Study the drawing (mm; zero at the part's minimum x, y, z) and answer. A direction names the side the tool comes from. Round coordinates to 2 decimals unless told otherwise and drop trailing zeros. Write each loop counter-clockwise with the first axis right and the second up, starting at its lowest first coordinate (ties: lowest second). Pieces come first, ordered by that corner, then holes. Notation, with made-up numbers: (42.5, -29) - (71.5, -29) arc R12 ccw to (71.5, -8) - close; hole circle Ø8 at (-13.5, 40). An arc over 180 degrees is marked (long way). Use one line per item in the form item = value. Start each with the question number.
1) The part is cut by section C-C, the plane z = 7. Give the vertices of the cut face in (x, y).
2) This flat-tipped pin is pushed along its axis until it touches: pin 1 (24 mm diameter, centred on x = 157.5, y = 37.5, fed in from +Z). Where does it stop, or does it pass through?
3) Consider line 1 along Y through (x, z) = (157.5, 11.75); line 2 along Z through (x, y) = (131, 12); line 3 along X through (y, z) = (37, 6). Determine where each line is inside the solid, lowest interval first. Write a range as from..to.
4) The part is cut by section A-A, the plane y = 37.5. Give the vertices of the cut face in (x, z), plus the area to 3 significant figures.
5) For a pull along Y with two mould halves and no side action, classify the marked faces 4, 5 and 6 as released by +Y, released by -Y, zero draft, split by the parting line, or undercut.
6) For the marked faces 1, 2 and 3, determine the directions among +Z, -Z, +X, -X, +Y, -Y from which every point of the face is accessible in a straight line to the end or side of a thin tool.
7) The part is cut by section D-D, the plane x = 157.5. Give the vertices of the cut face in (y, z), plus the area to 3 significant figures.
8) The part is cut by section B-B, the plane x = 74. Give the vertices of the cut face in (y, z).
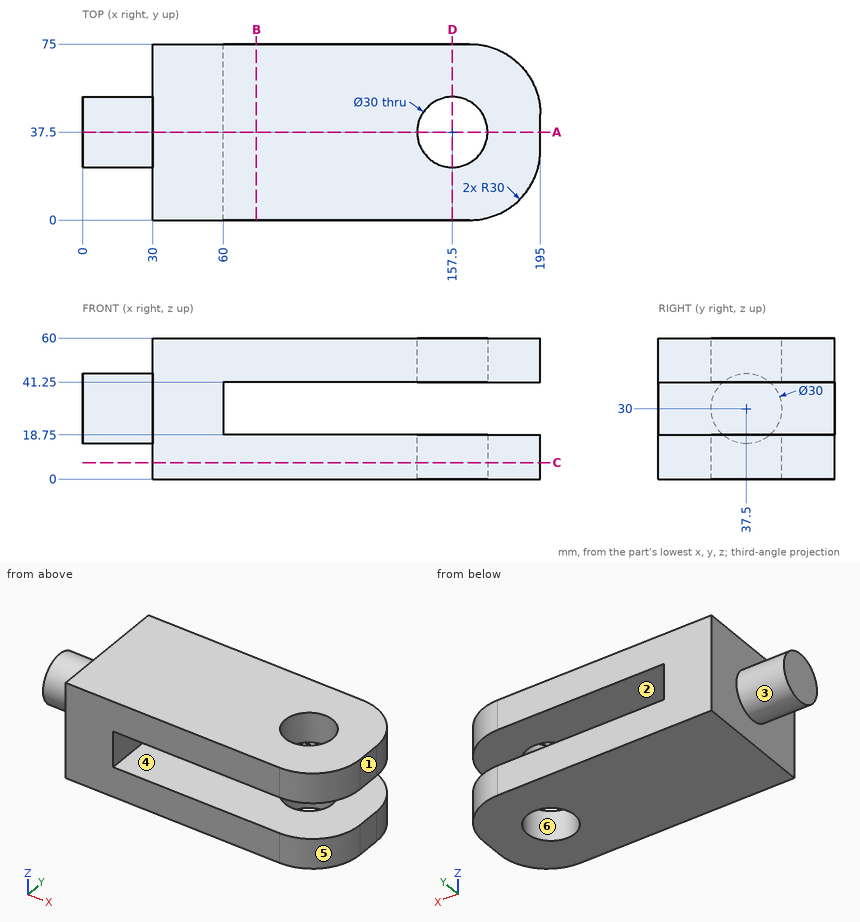
Geometry results:
q1.outline = (30, 0) - (165, 0) arc R30 ccw to (195, 30) - (195, 45) arc R30 ccw to (165, 75) - (30, 75) - close; hole circle Ø30 at (157.5, 37.5)
q2.pin_1 = through
q3.line_1 = 0..22.5, 52.5..75
q3.line_2 = 0..18.75, 41.25..60
q3.line_3 = 30..142.51, 172.49..195
q4.outline = (0, 15) - (30, 15) - (30, 0) - (142.5, 0) - (142.5, 18.75) - (60, 18.75) - (60, 41.25) - (142.5, 41.25) - (142.5, 60) - (30, 60) - (30, 45) - (0, 45) - close; (172.5, 0) - (195, 0) - (195, 18.75) - (172.5, 18.75) - close; (172.5, 41.25) - (195, 41.25) - (195, 60) - (172.5, 60) - close
q4.area = 6,640 mm2
q5.face_4 = zero draft
q5.face_5 = released by -Y
q5.face_6 = undercut
q6.face_1 = +Z, -Z, +X, +Y, -Y
q6.face_2 = +X, +Y, -Y
q6.face_3 = -X
q7.outline = (0, 0) - (22.5, 0) - (22.5, 18.75) - (0, 18.75) - close; (0, 41.25) - (22.5, 41.25) - (22.5, 60) - (0, 60) - close; (52.5, 0) - (75, 0) - (75, 18.75) - (52.5, 18.75) - close; (52.5, 41.25) - (75, 41.25) - (75, 60) - (52.5, 60) - close
q7.area = 1,690 mm2
q8.outline = (0, 0) - (75, 0) - (75, 18.75) - (0, 18.75) - close; (0, 41.25) - (75, 41.25) - (75, 60) - (0, 60) - close
